The model under review builds one solid part; all positions refer to its coordinate system, in mm. A direction names the side the tool comes from. Coordinates: 2 decimals unless noted, no trailing zeros. Loops run counter-clockwise (first coordinate to the right, second up) from the corner with the lowest first, then second, coordinate; pieces in that order, holes last. Notation, with made-up numbers: M -28,-19 L 26,-19 A27 ccw 26,5 Z; hole C 5.5,-11.5 d5. An arc over 180 degrees is marked long. Use CSV: the item, a comma, the result in double quotes. Start each with the question number.
from build123d import *

# Parameters (mm, degrees)
BOX014_W          = 23.6
BOX014_H          = 11.8
BOX014_DEPTH      = 10
BOX015_W          = 10.6
BOX015_H          = 4
BOX015_DEPTH      = 10
CYLINDER007_R     = 0.6
CYLINDER007_DEPTH = 10
ARRAY009_X_COUNT  = 2
ARRAY009_X_PITCH  = 29.6
ARRAY009_Y_COUNT  = 2
ARRAY009_Y_PITCH  = 17.8
BOX012_W          = 44.8
BOX012_H          = 33
BOX012_DEPTH      = 4
FILLET_R          = 5
FILLET003003_R    = 1.6


with BuildPart() as base_extraction_cube:
    # Box014 → Box014 (new body)
    with BuildSketch(Plane(origin=(6, 6, 0), x_dir=(1, 0, 0), z_dir=(0, 0, 1))):
        with Locations((11.8, 5.9)):
            Rectangle(BOX014_W, BOX014_H)
    extrude(amount=BOX014_DEPTH)


with BuildPart() as wire_channel:
    # Box015 → Box015 (new body)
    with BuildSketch(Plane(origin=(-4.6, 9.9, 0), x_dir=(1, 0, 0), z_dir=(0, 0, 1))):
        with Locations((5.3, 2)):
            Rectangle(BOX015_W, BOX015_H)
    extrude(amount=BOX015_DEPTH)


with BuildPart() as base_extract_fusion:
    # Cylinder007 → Cylinder007 (new body)
    with BuildSketch(Plane.XY):
        Circle(CYLINDER007_R)
    extrude(amount=CYLINDER007_DEPTH)

    # Array009 X: base extract fusion ×2


with BuildPart() as base_extract_fusion_1:
    add(base_extract_fusion.part)
    with Locations(*[(i * ARRAY009_X_PITCH, 0, 0) for i in range(1, ARRAY009_X_COUNT)]):
        add(base_extract_fusion.part)

    # Array009 Y: base extract fusion ×2


with BuildPart() as base_extract_fusion_2:
    add(base_extract_fusion_1.part)
    with Locations(*[(0, i * ARRAY009_Y_PITCH, 0) for i in range(1, ARRAY009_Y_COUNT)]):
        add(base_extract_fusion_1.part)


with BuildPart() as base_extract_fusion_3:
    # Array009 placement: moved
    add(base_extract_fusion_2.part.moved(Location((3, 3, 0))))

    # Fusion010: union base extraction cube, wire channel
    add(base_extraction_cube.part)
    add(wire_channel.part)


with BuildPart() as base_cut_fillet_no_ears:
    # Box012 → Box012 (new body)
    with BuildSketch(Plane(origin=(-4.6, -4.6, 0), x_dir=(1, 0, 0), z_dir=(0, 0, 1))):
        with Locations((22.4, 16.5)):
            Rectangle(BOX012_W, BOX012_H)
    extrude(amount=BOX012_DEPTH)

    # Fillet
    fillet_edges = [base_cut_fillet_no_ears.edges().sort_by_distance(p)[0] for p in [
        (-4.6, -4.6, 2),
        (-4.6, 28.4, 2),
        (40.2, -4.6, 2),
        (40.2, 28.4, 2),
    ]]
    fillet(fillet_edges, radius=FILLET_R)

    # Cut002003: cut base extract fusion
    add(base_extract_fusion_3.part, mode=Mode.SUBTRACT)

    # Fillet003003
    fillet003003_edges = [base_cut_fillet_no_ears.edges().sort_by_distance(p)[0] for p in [
        (-4.6, 9.9, 2),
        (6, 9.9, 2),
        (6, 13.9, 2),
        (-4.6, 13.9, 2),
    ]]
    fillet(fillet003003_edges, radius=FILLET003003_R)


solid = base_cut_fillet_no_ears.part
1. Add section C-C (x = 3). Write out the cut boundary in (y, z).
2. Add section D-D (z = 2.35). Write out the cut boundary in (x, y), plus the area to 3 significant figures.
3. For faces 1 (the cylindrical face through (-3.17, -3.1, 2.03)), 2 (the cylindrical face through (-4.12, 14.36, 2.03)), 3 (the flat face through (18, 17.8, 2)), list the 3-axis set-ups (+Z, -Z, +X, -X, +Y, -Y) from which the entire face can be reached by the end or side of a thin tool; tool diameter is ignored.
4. Add section A-A (x = 32.6). Write out the cut boundary in (y, z), plus the area to 3 significant figures.
5. Add section B-B (y = 17). Write out the cut boundary in (x, z).
6. Draft analysis for pull direction Y (two halves, no side actions). For faces 4 (the cylindrical face through (32, 3, 2)), 5 (the cylindrical face through (5.54, 14.38, 2.03)), 6 (the cylindrical face through (38.7, -3.17, 2.03)), 7 (the cylindrical face through (38.77, 26.9, 2.03)), state which applies: released by +Y, released by -Y, zero draft, split by the parting line, or undercut.
7. To check wall thickness, follow line 1 along X through (y, z) = (20.8, 1.65); line 2 along Y through (x, z) = (3, 2.7); line 3 along Y through (x, z) = (32.6, 2.7). State the ranges of each line that lie inside material, in increasing order.
8. Insertion check: pin 1 Ø1.1 at (x, y) = (32.6, 20.8) entering from +Z; pin 2 Ø1.2 at (y, z) = (11.5, 2.5) entering from -X. Each pin has a flat end and moves straight along its axis. Give the tip position at first contact, or say it passes through.
Solved:
1,outline,"M -4.6,0 L 2.4,0 L 2.4,4 L -4.6,4 Z; M 3.6,0 L 9.9,0 L 9.9,4 L 3.6,4 Z; M 13.9,0 L 20.2,0 L 20.2,4 L 13.9,4 Z; M 21.4,0 L 28.4,0 L 28.4,4 L 21.4,4 Z"
2,outline,"M -4.6,0.4 A5 ccw 0.4,-4.6 L 35.2,-4.6 A5 ccw 40.2,0.4 L 40.2,23.4 A5 ccw 35.2,28.4 L 0.4,28.4 A5 ccw -4.6,23.4 L -4.6,15.5 A1.6 ccw -3,13.9 L 4.4,13.9 A1.6 ccw 6,15.5 L 6,17.8 L 29.6,17.8 L 29.6,6 L 6,6 L 6,8.3 A1.6 ccw 4.4,9.9 L -3,9.9 A1.6 ccw -4.6,8.3 Z; hole C 3,3 d1.2; hole C 3,20.8 d1.2; hole C 32.6,3 d1.2; hole C 32.6,20.8 d1.2"
2,area,"1,130 mm^2"
3,face 1,"+Z, -Z, -X, -Y"
3,face 2,"+Z, -Z, -X"
3,face 3,"+Z, -Z"
4,outline,"M -4.6,0 L 2.4,0 L 2.4,4 L -4.6,4 Z; M 3.6,0 L 20.2,0 L 20.2,4 L 3.6,4 Z; M 21.4,0 L 28.4,0 L 28.4,4 L 21.4,4 Z"
4,area,"122 mm^2"
5,outline,"M -4.6,0 L 6,0 L 6,4 L -4.6,4 Z; M 29.6,0 L 40.2,0 L 40.2,4 L 29.6,4 Z"
6,face 4,"undercut"
6,face 5,"undercut"
6,face 6,"released by -Y"
6,face 7,"released by +Y"
7,line 1,"x = -4.6 to 2.4, 3.6 to 32, 33.2 to 40.2"
7,line 2,"y = -4.6 to 2.4, 3.6 to 9.9, 13.9 to 20.2, 21.4 to 28.4"
7,line 3,"y = -4.6 to 2.4, 3.6 to 20.2, 21.4 to 28.4"
8,pin 1,"passes through"
8,pin 2,"stops at x = 29.6"
